Check sheet for the drawn part. Datum: minimum x, y, z corner. Units: mm. Coordinates: 2 decimals unless noted, no trailing zeros. Order: outer loops, then holes, each group sorted by start corner. A loop starts at its lowest first (then second) coordinate and runs counter-clockwise, first axis right, second up.
1. Gauge pin test, flat ends, axial feed: pin 1 Ø8 at (x, y) = (54.5, 119.5) entering from +Z; pin 2 Ø6 at (y, z) = (75.5, 8.5) entering from -X; pin 3 Ø20.5 at (x, y) = (47, 75) entering from +Z. Record the tip position at first contact, or that the pin passes through.
2. Thickness scan on line 1 (Y direction, x = 29, z = 17.5); line 2 (Z direction, x = 85, y = 41); line 3 (Z direction, x = 55.5, y = 83). Record the ranges inside material, lowest first.
3. Cross-section at A-A (z = 10.5). Count the separate pieces of the cut face and the enclosed holes in it, then the cut area to 3 significant figures.
4. Cross-section at C-C (y = 68). Enter the section's corners in (x, z).
5. Cross-section at B-B (x = 39.5). Enter the section's corners in (y, z).
6. Cross-section at D-D (y = 129.5). Enter the section's corners in (x, z).
7. Draft check along Y on the marked faces 1 and 2. Enter one of: released by +Y, released by -Y, zero draft, split by the parting line, or undercut.
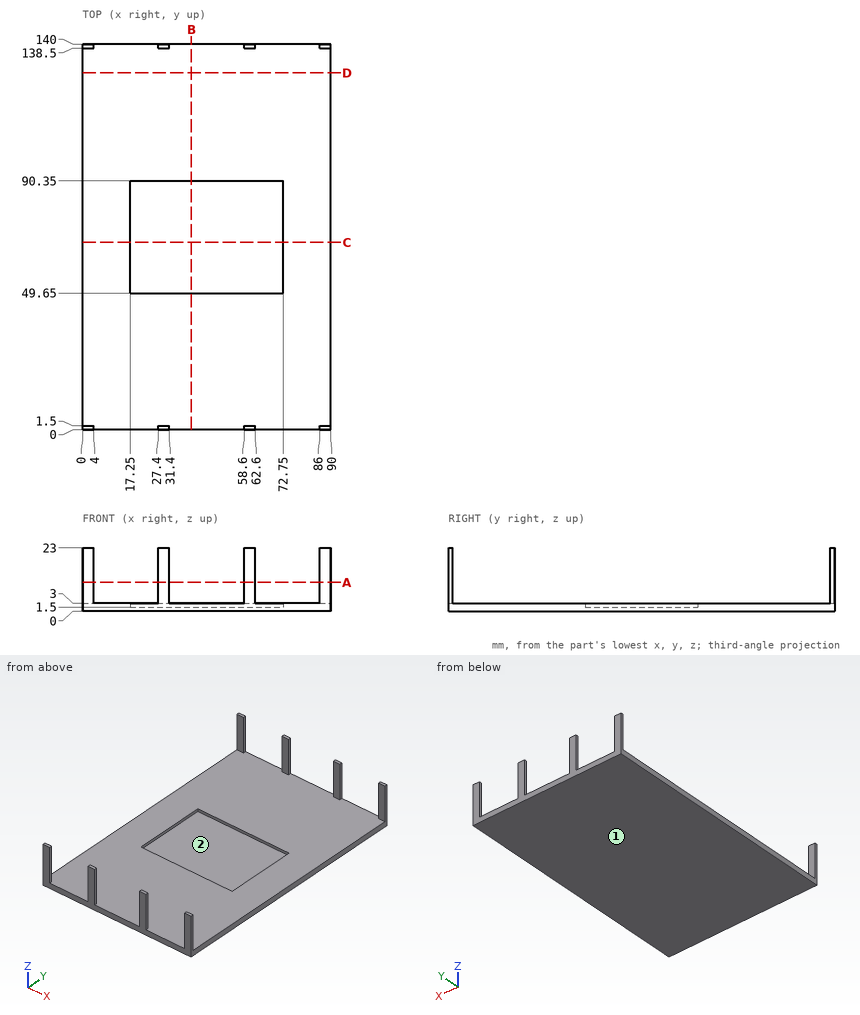
Data:
1. pin 1: stops at z = 3
1. pin 2: passes through
1. pin 3: stops at z = 1.5
2. line 1: y = 0 to 1.5, 138.5 to 140
2. line 2: z = 0 to 3
2. line 3: z = 0 to 1.5
3. separate pieces: 8
3. enclosed holes: 0
3. area: 48.0 mm2
4. outline: (0, 0) - (90, 0) - (90, 3) - (72.75, 3) - (72.75, 1.5) - (17.25, 1.5) - (17.25, 3) - (0, 3) - close
5. outline: (0, 0) - (140, 0) - (140, 3) - (90.35, 3) - (90.35, 1.5) - (49.65, 1.5) - (49.65, 3) - (0, 3) - close
6. outline: (0, 0) - (90, 0) - (90, 3) - (0, 3) - close
7. face 1: zero draft
7. face 2: undercut
